Print and shaded views of the part. All mm, measured from the part's lowest x, y and z. Give positions to 0.01 mm unless a question says otherwise; leave off trailing zeros. Loops run counter-clockwise (first coordinate to the right, second up) from the corner with the lowest first, then second, coordinate; pieces in that order, holes last.
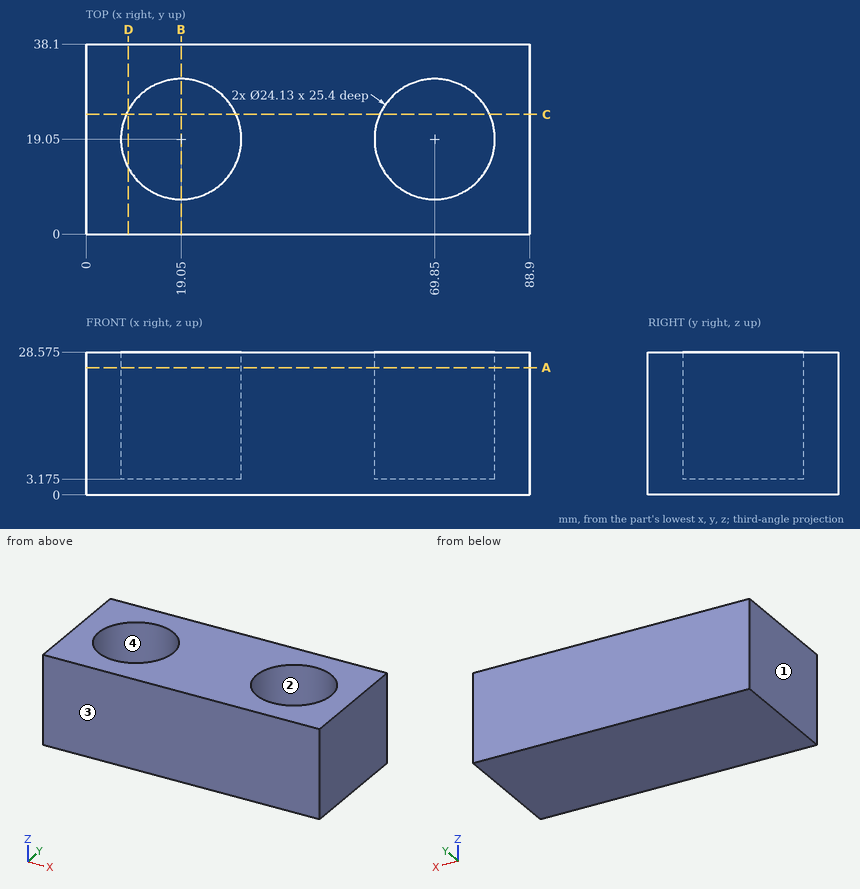
1. Saw through at D-D, the plane x = 8.5. List the corners of the cut face in (y, z) (3 decimals).
Responses:
outline: (0, 0) - (38.1, 0) - (38.1, 28.575) - (24.903, 28.575) - (24.903, 3.175) - (13.197, 3.175) - (13.197, 28.575) - (0, 28.575) - close
2. Saw through at A-A, the plane z = 25.5. List the corners of the cut face in (x, y) (3 decimals).
Responses:
outline: (0, 0) - (88.9, 0) - (88.9, 38.1) - (0, 38.1) - close; hole circle Ø24.13 at (19.05, 19.05); hole circle Ø24.13 at (69.85, 19.05)
3. Saw through at B-B, the plane x = 19.05. List the corners of the cut face in (y, z) (3 decimals).
Responses:
outline: (0, 0) - (38.1, 0) - (38.1, 28.575) - (31.115, 28.575) - (31.115, 3.175) - (6.985, 3.175) - (6.985, 28.575) - (0, 28.575) - close
4. Pull direction X, two halves, no side cores. Call the marked faces 1, 2, 3 and 4: released by +X, released by -X, zero draft, split by the parting line, or undercut.
Responses:
face 1: released by -X
face 2: undercut
face 3: zero draft
face 4: undercut
5. Probe line 1 along Y through (x, z) = (19.05, 22.5) (3 decimals); line 2 along X through (y, z) = (24, 25.75); line 3 along X through (y, z) = (26.5, 19.25). List the from-to ranges inside material, lowest first.
Responses:
line 1: y = 0 to 6.985, 31.115 to 38.1
line 2: x = 0 to 8.05, 30.05 to 58.85, 80.85 to 88.9
line 3: x = 0 to 9.56, 28.54 to 60.36, 79.34 to 88.9
6. Saw through at C-C, the plane y = 24. List the corners of the cut face in (x, z) (3 decimals), and give its area (3 significant figures).
Responses:
outline: (0, 0) - (88.9, 0) - (88.9, 28.575) - (80.853, 28.575) - (80.853, 3.175) - (58.847, 3.175) - (58.847, 28.575) - (30.053, 28.575) - (30.053, 3.175) - (8.047, 3.175) - (8.047, 28.575) - (0, 28.575) - close
area: 1,420 mm2
7. Drop flat-ended pins along their axis: pin 1 (8 mm diameter, centred on x = 74.5, z = 24.5, fed in from -Y); pin 2 (1 mm diameter, centred on x = 22.5, y = 22, fed in from +Z) (3 decimals). Give the stop position or say it passes through.
Responses:
pin 1: stops at y = 0
pin 2: stops at z = 3.175
